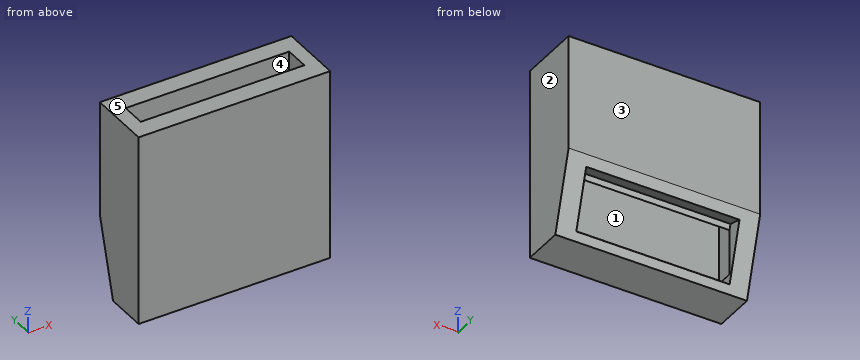
```python
from build123d import *

# Parameters (mm, degrees)
F0_W     = 31.75
F0_H     = 10.414
F1_DEPTH = 31.75
F2_W     = 27.1145
F2_H     = 4.064
F3_DEPTH = 28.575
F4_SIZE2 = 3.556
F4_SIZE  = 12.7
F5_W     = 25.4
F5_H     = 9.839699956
F6_DEPTH = 2.5146


with BuildPart() as f1:
    # F0 (on Top) → F1 (new body)
    with BuildSketch(Plane.XY):
        Rectangle(F0_W, F0_H)
    extrude(amount=F1_DEPTH)

    # F2 (on face) → F3 (cut)
    with BuildSketch(Plane.XY.offset(31.75)):
        Rectangle(F2_W, F2_H)
    extrude(amount=-F3_DEPTH, mode=Mode.SUBTRACT)

    # F4
    f4_edges = [f1.edges().sort_by_distance(p)[0] for p in [
        (0, 5.207, 0),
    ]]
    f4_side = f1.faces().sort_by_distance((0, 5.207, 15.875))[0]
    chamfer(f4_edges, length=F4_SIZE, length2=F4_SIZE2, reference=f4_side)

    # F5 (on face) → F6 (cut)
    with BuildSketch(Plane(origin=(0, 1.5309718101, -0.4286721068), x_dir=(-1, 0, 0), z_dir=(0, 0.9629640197, -0.2696299255))):
        with Locations((0.0492152758, 6.8765128963)):
            Rectangle(F5_W, F5_H)
    extrude(amount=-F6_DEPTH, mode=Mode.SUBTRACT)


solid = f1.part
```
Could you check a few things on this model? Use its own coordinates, in mm. Face numbers are marked on the shaded views. A direction names the side the tool comes from. Coordinates: 2 decimals unless noted, no trailing zeros. Write each loop counter-clockwise with the first axis right and the second up, starting at its lowest first coordinate (ties: lowest second). Pieces come first, ordered by that corner, then holes. Notation, with made-up numbers: (-10.75, 76) - (47.25, 76) arc R25 cw to (47.25, 109) - close; hole circle Ø4 at (3, 55.5). An arc over 180 degrees is marked (long way). Use a Markdown table: item, result.
Q1. Imagine slicing it at D-D (z = 9). List the corners of the cut face in (x, y) for me (3 decimals).
Geometry check:
| item | result |
|---|---|
| outline | (-15.875, -5.207) - (15.875, -5.207) - (15.875, 4.171) - (12.651, 4.171) - (12.651, 2.032) - (13.557, 2.032) - (13.557, -2.032) - (-13.557, -2.032) - (-13.557, 2.032) - (-12.749, 2.032) - (-12.749, 4.171) - (-15.875, 4.171) - close |
Q2. Imagine slicing it at A-A (z = 24). List the corners of the cut face in (x, y) for me (3 decimals).
Geometry check:
| item | result |
|---|---|
| outline | (-15.875, -5.207) - (15.875, -5.207) - (15.875, 5.207) - (-15.875, 5.207) - close; hole (-13.557, -2.032) - (13.557, -2.032) - (13.557, 2.032) - (-13.557, 2.032) - close |
Q3. I'm going to push a flat-ended pin straight in: pin 1 Ø1.2 at (x, y) = (5.5, -1) entering from +Z (3 decimals). Where does the tip first touch, or does it pass through?
Geometry check:
| item | result |
|---|---|
| pin 1 | stops at z = 3.175 |
Q4. Which directions (+Z, -Z, +X, -X, +Y, -Y) give clear straight access to the entire face, cutting with the end or side of a thin tool? Please do the marked faces 1 and 2.
Geometry check:
| item | result |
|---|---|
| face 1 | +Z |
| face 2 | +Z, -Z, +X, +Y, -Y |
Q5. Thinking about a two-plate mould opening in Y: for the marked faces 3, 4 and 5, which applies, +Y half, -Y half, draft (parallel to the pull), parting line (faces both ways), or undercut?
Geometry check:
| item | result |
|---|---|
| face 3 | +Y half |
| face 4 | undercut |
| face 5 | draft |
Q6. Imagine slicing it at C-C (y = 0.5). List the corners of the cut face in (x, z) for me (3 decimals).
Geometry check:
| item | result |
|---|---|
| outline | (-15.875, 0) - (15.875, 0) - (15.875, 31.75) - (13.557, 31.75) - (13.557, 3.175) - (12.651, 3.175) - (12.651, 1.892) - (-12.749, 1.892) - (-12.749, 3.175) - (-13.557, 3.175) - (-13.557, 31.75) - (-15.875, 31.75) - close |
Q7. Imagine slicing it at B-B (x = -8). List the corners of the cut face in (y, z) for me (3 decimals).
Geometry check:
| item | result |
|---|---|
| outline | (-5.207, 0) - (1.651, 0) - (2.059, 1.456) - (-0.363, 2.134) - (-0.071, 3.175) - (-2.032, 3.175) - (-2.032, 31.75) - (-5.207, 31.75) - close; (2.032, 10.687) - (2.29, 11.609) - (4.712, 10.931) - (5.207, 12.7) - (5.207, 31.75) - (2.032, 31.75) - close |
Q8. Please list where these lines run through material, in increasing order: L1, parallel to Y at x = 7, z = 30.5; L2, parallel to X at y = -0.5, z = 12.5 (3 decimals); L3, parallel to X at y = 2.5, z = 7 (3 decimals).
Geometry check:
| item | result |
|---|---|
| L1 | y = -5.21 to -2.03, 2.03 to 5.21 |
| L2 | x = -15.875 to -13.557, 13.557 to 15.875 |
| L3 | x = -15.875 to -12.749, 12.651 to 15.875 |
